Design review of the part built by this model. Coordinates are the model's own, in mm. Coordinates: 2 decimals unless noted, no trailing zeros. Loops run counter-clockwise (first coordinate to the right, second up) from the corner with the lowest first, then second, coordinate; pieces in that order, holes last. Notation, with made-up numbers: M 85.25,-19 L 97.25,-19 A17 cw 97.25,-7 Z; hole C 19,76 d3. An arc over 180 degrees is marked long. Answer as a JSON object with one key per item and string values. Group by question number.
1. Consider section A-A (z = -0.5). State the section outline as (x, y) points.
2. Insertion check: pin 1 (3.5 mm diameter, centred on x = 0, y = 67.23, fed in from -Z). The pin has a flat end and moves straight along its axis. Give the tip position at first contact, or say it passes through.
3. Draft analysis for pull direction X (two halves, no side actions). For faces 1 (the cylindrical face through (-0.412, -65.374, 0.014)), 2 (the cylindrical face through (-2.24, -70.09, 0.01)), 3 (the cylindrical face through (2.2, -70.13, 0.01)), state which applies: +X half, -X half, draft (parallel to the pull), parting line (faces both ways), or undercut.
4. To check wall thickness, follow probe 1 along Y at (x, z) = (0, -0.05); probe 2 along Y at (x, z) = (0.65, -0.5); probe 3 along Y at (x, z) = (-1.6, -0.25). State the ranges of each line that lie inside material, in increasing order.
from build123d import *

# Parameters (mm, degrees)
F0_W          = 5.9313117526
F0_H          = 1.9345532637
F1_DEPTH      = 70.8533
F1_DEPTH_BACK = 70.8533
F2_R          = 2.54
F3_R          = 1.9022356475
F4_DEPTH      = 2.3622
F5_R          = 1.0755010134
F6_DEPTH      = 2.01676


# Not quite as in the source:
# - a pattern or mirror of a feature is missing from the dataset's text; its kind, count and spacing are read off the source's solid


with BuildPart() as f1:
    # F0 (on Front) → F1 (new body, two sides)
    with BuildSketch(Plane.XZ) as f1_sk:
        Rectangle(F0_W, F0_H)
    extrude(amount=F1_DEPTH)
    extrude(f1_sk.sketch, amount=-F1_DEPTH_BACK)

    # F2
    f2_edges = [f1.edges().sort_by_distance(p)[0] for p in [
        (2.965656, -70.8533, 0),
        (-2.965656, -70.8533, 0),
        (2.965656, 70.8533, 0),
        (-2.965656, 70.8533, 0),
    ]]
    fillet(f2_edges, radius=F2_R)

    # F3 (on face) → F4 (cut)
    with BuildSketch(Plane.XY.offset(0.9672766319)):
        with Locations((0, 67.2314763069)):
            Circle(F3_R)
    f4 = extrude(amount=-F4_DEPTH, mode=Mode.SUBTRACT)

    # F4_copies: F4 across plane
    add(f4.mirror(Plane(origin=(0, 0, 0), x_dir=(0, 0, -1), z_dir=(0, -1, 0))), mode=Mode.SUBTRACT)

    # F5 (on face) → F6 (cut)
    with BuildSketch(Plane.XY.offset(0.9672766319)):
        Circle(F5_R)
    extrude(amount=-F6_DEPTH, mode=Mode.SUBTRACT)


solid = f1.part
Findings below:
{
 "1": {"outline": "M -2.97,-68.31 A2.54 ccw -0.43,-70.85 L 0.43,-70.85 A2.54 ccw 2.97,-68.31 L 2.97,68.31 A2.54 ccw 0.43,70.85 L -0.43,70.85 A2.54 ccw -2.97,68.31 Z; hole C 0,-67.23 d3.8; hole C 0,67.23 d3.8; hole C 0,0 d2.15"},
 "2": {"pin 1": "passes through"},
 "3": {"face 1": "undercut", "face 2": "-X half", "face 3": "+X half"},
 "4": {"probe 1": "y = -70.85 to -69.13, -65.33 to -1.08, 1.08 to 65.33, 69.13 to 70.85", "probe 2": "y = -70.84 to -69.02, -65.44 to -0.86, 0.86 to 65.44, 69.02 to 70.84", "probe 3": "y = -70.57 to -68.26, -66.2 to 66.2, 68.26 to 70.57"}
}
